```python
from build123d import *

# Parameters (mm, degrees)
SKETCH1_W           = 30.95625
SKETCH1_H           = 47.625
SKETCH1_R           = 7.9121
BOSS_EXTRUDE1_DEPTH = 7.540625
SKETCH2_W           = 30.95625
SKETCH2_H           = 22.1996
SKETCH2_R           = 7.9121
BOSS_EXTRUDE2_DEPTH = 8.334375


with BuildPart() as part:
    # Sketch1 → Boss-Extrude1 (new body)
    with BuildSketch(Plane(origin=(0, 0, 0), x_dir=(1, 0, 0), z_dir=(0, 1, 0))):
        Rectangle(SKETCH1_W, SKETCH1_H)
        Circle(SKETCH1_R, mode=Mode.SUBTRACT)
    extrude(amount=BOSS_EXTRUDE1_DEPTH)

    # Sketch2 → Boss-Extrude2 (add)
    with BuildSketch(Plane(origin=(0, 7.540625, 0), x_dir=(1, 0, 0), z_dir=(0, 1, 0))):
        Rectangle(SKETCH2_W, SKETCH2_H)
        Circle(SKETCH2_R, mode=Mode.SUBTRACT)
    extrude(amount=BOSS_EXTRUDE2_DEPTH)


solid = part.part
```
For this review, take the finished solid that the model builds, in its own axes (mm). A direction names the side the tool comes from. Coordinates: 2 decimals unless noted, no trailing zeros. Order: outer loops, then holes, each group sorted by start corner. A loop starts at its lowest first (then second) coordinate and runs counter-clockwise, first axis right, second up. Notation, with made-up numbers: (59.25, 78.5) -> (75.25, 78.5) arc R26 ccw to (75.25, 116.5) -> close; hole circle Ø8 at (46.25, -8.5). An arc over 180 degrees is marked (long way). Use CSV: the item, a comma, the result in double quotes. Start each with the question number.
Item 1: We need section B-B, the plane z = 0. Give the boundary of the cut face in (x, y) (3 decimals), then the cut area to 3 significant figures.
Item 2: Draft analysis for pull direction Z (two halves, no side actions). For faces 4 (the face through (0, 4, -23.812)), 5 (the face through (-1.715, 7.826, 7.724)), 6 (the face through (0, 4, 23.812)), 7 (the face through (-7, 0, -6)), state which applies: pulls with the +Z half, pulls with the -Z half, needs draft (parallel to the pull), parting line crosses it, or undercut.
Item 3: We need section A-A, the plane x = 0. Give the boundary of the cut face in (y, z) (1 decimal).
Item 4: For faces 1 (the face through (15.478, 6, 0)), 2 (the face through (0, 12, 11.1)), 3 (the face through (0, 7.541, -18)), list the 3-axis set-ups (+Z, -Z, +X, -X, +Y, -Y) from which the entire face can be reached by the end or side of a thin tool; tool diameter is ignored.
Item 5: We need section C-C, the plane x = 10. Give the boundary of the cut face in (y, z) (1 decimal), then the cut area to 3 significant figures.
Item 6: Insertion check: pin 1 (4 mm diameter, centred on x = 2, y = 12, fed in from -Z); pin 2 (6.5 mm diameter, centred on x = -7, z = 15, fed in from +Y). Each pin has a flat end and moves straight along its axis. Give the tip position at first contact, or say it passes through.
Item 7: Wall thickness on probe 1 along Z at (x, y) = (0, 8.5); probe 2 along X at (y, z) = (12.5, 0); probe 3 along Z at (x, y) = (0, 6): over which ranges is each line inside the solid? List them lowest first.
Item 8: We need section D-D, the plane y = 13.5. Give the boundary of the cut face in (x, z), then the cut area to 3 significant figures.
Derived:
1,outline,"(-15.478, 0) -> (-7.912, 0) -> (-7.912, 15.875) -> (-15.478, 15.875) -> close; (7.912, 0) -> (15.478, 0) -> (15.478, 15.875) -> (7.912, 15.875) -> close"
1,area,"240 mm^2"
2,face 4,"pulls with the -Z half"
2,face 5,"undercut"
2,face 6,"pulls with the +Z half"
2,face 7,"needs draft"
3,outline,"(0, -23.8) -> (7.5, -23.8) -> (7.5, -11.1) -> (15.9, -11.1) -> (15.9, -7.9) -> (0, -7.9) -> close; (0, 7.9) -> (15.9, 7.9) -> (15.9, 11.1) -> (7.5, 11.1) -> (7.5, 23.8) -> (0, 23.8) -> close"
4,face 1,"+Z, -Z, +X, +Y, -Y"
4,face 2,"+Z, +X, -X, +Y"
4,face 3,"-Z, +X, -X, +Y"
5,outline,"(0, -23.8) -> (7.5, -23.8) -> (7.5, -11.1) -> (15.9, -11.1) -> (15.9, 11.1) -> (7.5, 11.1) -> (7.5, 23.8) -> (0, 23.8) -> close"
5,area,"544 mm^2"
6,pin 1,"stops at z = -11.1"
6,pin 2,"stops at y = 7.54"
7,probe 1,"z = -11.1 to -7.91, 7.91 to 11.1"
7,probe 2,"x = -15.48 to -7.91, 7.91 to 15.48"
7,probe 3,"z = -23.81 to -7.91, 7.91 to 23.81"
8,outline,"(-15.48, -11.1) -> (15.48, -11.1) -> (15.48, 11.1) -> (-15.48, 11.1) -> close; hole circle Ø15.82 at (0, 0)"
8,area,"491 mm^2"
